The figure shows three views and two pictorial views of one solid part (mm, origin at its lowest corner). Answer the questions. Give positions to 0.01 mm unless a question says otherwise; leave off trailing zeros. Order: outer loops, then holes, each group sorted by start corner. A loop starts at its lowest first (then second) coordinate and runs counter-clockwise, first axis right, second up. Notation, with made-up numbers: M 59,87 L 96,87 A6 ccw 96,93 Z; hole C -29.75,24.5 d7. An arc over 180 degrees is marked long. Write item = value, one per line. Start each with the question number.
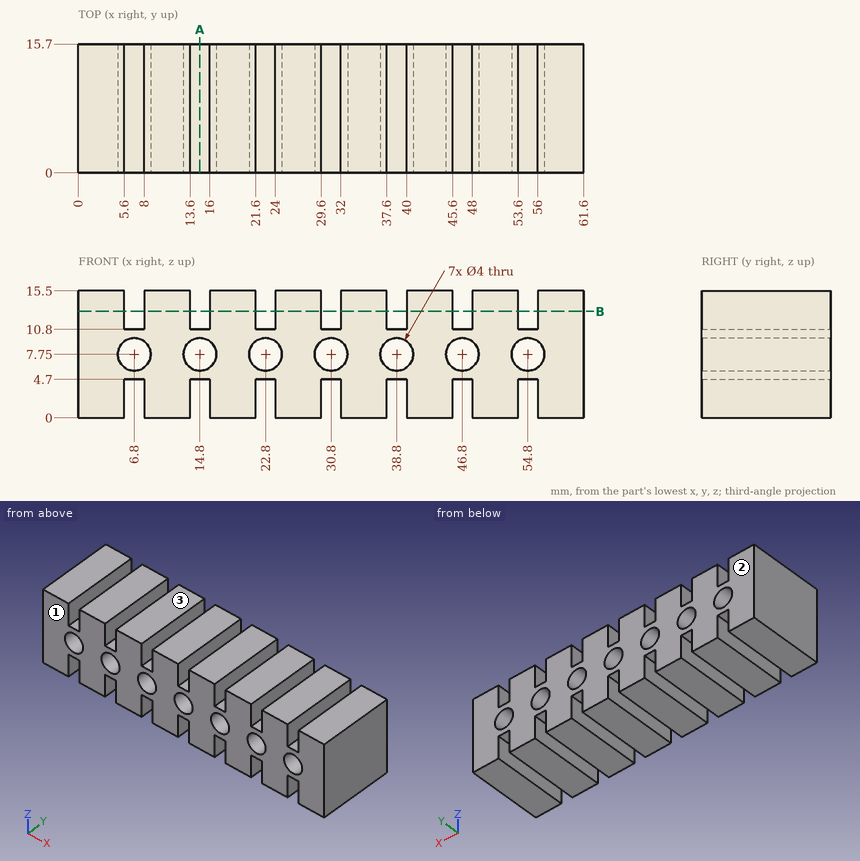
1) For a pull along Y with two mould halves and no side action, classify the marked faces 1, 2 and 3 as pulls with the +Y half, pulls with the -Y half, needs draft (parallel to the pull), parting line crosses it, or undercut.
2) Find the intervals of material crossed by probe 1 along Z at (x, y) = (54.8, 9.5); probe 2 along Z at (x, y) = (46, 7.25), in increasing order. Write a range as [from, to].
3) Find section B-B on z = 13. Count the separate pieces of the cut face and the enclosed holes in it, plus the area to 3 significant figures.
4) Find section A-A on x = 14.8. Determine the outline of the cut face in (y, z).
5) This flat-tipped pin is pushed along its axis until it touches: P1, Ø1, axis at y = 6.5, z = 11.5, coming from the -X side. Where does it stop, or does it pass through?
Numbers:
q1.face_1 = pulls with the -Y half
q1.face_2 = pulls with the +Y half
q1.face_3 = needs draft
q2.probe_1 = [4.7, 5.75], [9.75, 10.8]
q2.probe_2 = [4.7, 5.92], [9.58, 10.8]
q3.separate_pieces = 8
q3.enclosed_holes = 0
q3.area = 703 mm2
q4.outline = M 0,4.7 L 15.7,4.7 L 15.7,5.75 L 0,5.75 Z; M 0,9.75 L 15.7,9.75 L 15.7,10.8 L 0,10.8 Z
q5.P1 = 0
